Could you check a few things on this model? Use its own coordinates, in mm. Face numbers are marked on the shaded views. A direction names the side the tool comes from. Give positions to 0.01 mm unless a question says otherwise; leave off trailing zeros. Order: outer loops, then holes, each group sorted by start corner. A loop starts at its lowest first (then second) coordinate and runs counter-clockwise, first axis right, second up.
from build123d import *

# Parameters (mm, degrees)
SKETCH_1_W          = 65
SKETCH_1_H          = 65
SKETCH_1_R          = 2.6
SKETCH_1_R_2        = 19.1
EXTRUDE_1_DEPTH     = 1
SKETCH_2_W          = 65
SKETCH_2_H          = 1
EXTRUDE_2_DEPTH     = 67
CUT_EXTRUDE_1_DEPTH = 99.874920986


with BuildPart() as part:
    # 草图1 → 凸台-拉伸1 (new body)
    with BuildSketch(Plane(origin=(0, 0, 0), x_dir=(1, 0, 0), z_dir=(0, 1, 0))):
        Rectangle(SKETCH_1_W, SKETCH_1_H)
        with Locations(Location((-23.57, 23.57, 0), (0, 0, 270))):
            Circle(SKETCH_1_R, mode=Mode.SUBTRACT)
        with Locations(Location((23.57, 23.57, 0), (0, 0, 90))):
            Circle(SKETCH_1_R, mode=Mode.SUBTRACT)
        with Locations(Location((23.57, -23.57, 0), (0, 0, 270))):
            Circle(SKETCH_1_R, mode=Mode.SUBTRACT)
        with Locations(Location((-23.57, -23.57, 0), (0, 0, 90))):
            Circle(SKETCH_1_R, mode=Mode.SUBTRACT)
        with Locations(Location((0, 0, 0), (0, 0, 270))):
            Circle(SKETCH_1_R_2, mode=Mode.SUBTRACT)
    extrude(amount=EXTRUDE_1_DEPTH)

    # 草图2 → 凸台-拉伸2 (add)
    with BuildSketch(Plane(origin=(0, 1, 0), x_dir=(1, 0, 0), z_dir=(0, 1, 0))):
        with Locations((0, -32)):
            Rectangle(SKETCH_2_W, SKETCH_2_H)
    extrude(amount=EXTRUDE_2_DEPTH)

    # 草图3 → 切除-拉伸1 (cut, through all)
    with BuildSketch(Plane(origin=(0, 0, 31.5), x_dir=(-1, 0, 0), z_dir=(0, 0, -1))):
        with BuildLine():
            Line((-17.9, 58), (-17.9, 16))
            ThreePointArc((-17.9, 16), (-20, 13.9), (-22.1, 16))
            Line((-22.1, 16), (-22.1, 58))
            ThreePointArc((-22.1, 58), (-20, 60.1), (-17.9, 58))
        make_face()
        with BuildLine():
            Line((17.9, 58), (17.9, 16))
            ThreePointArc((17.9, 16), (20, 13.9), (22.1, 16))
            Line((22.1, 16), (22.1, 58))
            ThreePointArc((22.1, 58), (20, 60.1), (17.9, 58))
        make_face()
    extrude(amount=-CUT_EXTRUDE_1_DEPTH, mode=Mode.SUBTRACT)


solid = part.part
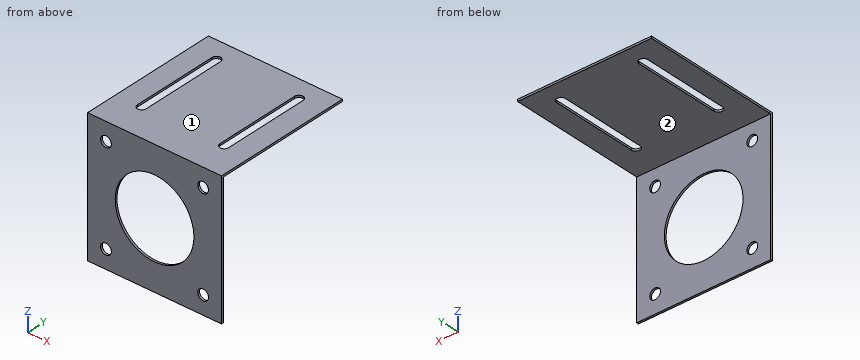
Item 1: For pin 1 (8.5 mm diameter, centred on x = 23.57, z = 23.57, fed in from +Y); pin 2 (1 mm diameter, centred on x = -15.5, z = 25, fed in from -Y); pin 3 (3 mm diameter, centred on x = -23.57, z = -23.57, fed in from +Y); pin 4 (19.5 mm diameter, centred on x = -3, y = 26, fed in from -Z), each with a flat end and sliding along its axis, tell me the tip position at first contact or that it passes through.
Findings:
pin 1: stops at y = 1
pin 2: stops at y = 0
pin 3: passes through
pin 4: stops at z = 31.5
Item 2: Imagine slicing it at C-C on z = 23.57. List the corners of the cut face in (x, y) for me.
Findings:
outline: (-32.5, 0) - (-26.17, 0) - (-26.17, 1) - (-32.5, 1) - close; (-20.97, 0) - (20.97, 0) - (20.97, 1) - (-20.97, 1) - close; (26.17, 0) - (32.5, 0) - (32.5, 1) - (26.17, 1) - close
Item 3: Imagine slicing it at A-A on x = -23.57. List the corners of the cut face in (y, z) for me, then the cut area to 3 significant figures.
Findings:
outline: (0, -32.5) - (1, -32.5) - (1, -26.17) - (0, -26.17) - close; (0, -20.97) - (1, -20.97) - (1, 20.97) - (0, 20.97) - close; (0, 26.17) - (1, 26.17) - (1, 31.5) - (68, 31.5) - (68, 32.5) - (0, 32.5) - close
area: 122 mm2
Item 4: Imagine slicing it at D-D on x = 4. List the corners of the cut face in (y, z) for me, then the cut area to 3 significant figures.
Findings:
outline: (0, -32.5) - (1, -32.5) - (1, -18.68) - (0, -18.68) - close; (0, 18.68) - (1, 18.68) - (1, 31.5) - (68, 31.5) - (68, 32.5) - (0, 32.5) - close
area: 94.6 mm2
Item 5: For the marked faces 1 and 2, which set-ups out of +Z, -Z, +X, -X, +Y, -Y let a thin tool reach every point of the face, with its end or its side?
Findings:
face 1: +Z, +X, -X, +Y, -Y
face 2: -Z, +X, -X, +Y
Item 6: Imagine slicing it at B-B on y = 57. List the corners of the cut face in (x, z) for me, then the cut area to 3 significant figures.
Findings:
outline: (-32.5, 31.5) - (-22.1, 31.5) - (-22.1, 32.5) - (-32.5, 32.5) - close; (-17.9, 31.5) - (17.9, 31.5) - (17.9, 32.5) - (-17.9, 32.5) - close; (22.1, 31.5) - (32.5, 31.5) - (32.5, 32.5) - (22.1, 32.5) - close
area: 56.6 mm2
Item 7: Please list where these lines run through material, in increasing order: line 1 along X through (y, z) = (0.45, 23.57); line 2 along Z through (x, y) = (-5.5, 13.5); line 3 along Y through (x, z) = (-25, 21).
Findings:
line 1: x = -32.5 to -26.17, -20.97 to 20.97, 26.17 to 32.5
line 2: z = 31.5 to 32.5
line 3: y = 0 to 1
